from build123d import *

# Parameters (mm, degrees)
SKETCH_W     = 46
SKETCH_H     = 43.5
SKETCH_R     = 18.2
PAD_DEPTH    = 5
SKETCH006_R  = 1.5
POCKET_DEPTH = 5.001
FILLET_R     = 5
FILLET001_R  = 5


with BuildPart() as part:
    # Sketch → Pad (new body)
    with BuildSketch(Plane.YZ):
        with Locations((20, 15.75)):
            Rectangle(SKETCH_W, SKETCH_H)
        with Locations((18.5, 15.75)):
            Circle(SKETCH_R, mode=Mode.SUBTRACT)
    extrude(amount=PAD_DEPTH)

    # Sketch006 → Pocket (cut, through all)
    with BuildSketch(Plane.YZ.offset(5)):
        with Locations((3, 34.5)):
            Circle(SKETCH006_R)
        with Locations((34, 34.5)):
            Circle(SKETCH006_R)
        with Locations((40, 15.75)):
            Circle(SKETCH006_R)
        with Locations((34, -3)):
            Circle(SKETCH006_R)
        with Locations((3, -3)):
            Circle(SKETCH006_R)
    extrude(amount=-POCKET_DEPTH, mode=Mode.SUBTRACT)

    # Fillet
    fillet_edges = [part.edges().sort_by_distance(p)[0] for p in [
        (2.5, 43, -6),
        (2.5, -3, -6),
    ]]
    fillet(fillet_edges, radius=FILLET_R)

    # Fillet001
    fillet001_edges = [part.edges().sort_by_distance(p)[0] for p in [
        (2.5, 43, 37.5),
        (2.5, -3, 37.5),
    ]]
    fillet(fillet001_edges, radius=FILLET001_R)


solid = part.part
Build history of the part. All positions in model axes, mm. Round coordinates to 2 decimals unless told otherwise and drop trailing zeros. Write each loop counter-clockwise with the first axis right and the second up, starting at its lowest first coordinate (ties: lowest second). Pieces come first, ordered by that corner, then holes. Notation, with made-up numbers: (-27, 39.5) -> (27, 39.5) arc R24 ccw to (27, 52.5) -> close; hole circle Ø4 at (-8, -16). An arc over 180 degrees is marked (long way). Use one line per item in the form item = value.
Q1. Drill centre lines: L1, parallel to Z at x = 3.7, y = 18.5; L2, parallel to Z at x = 3.95, y = 3; L3, parallel to Y at x = 0.2, z = 16. Where is each one in solid material? Low to high.
Conclusion:
L1 = -6 to -2.45, 33.95 to 37.5
L2 = -6 to -4.5, -1.5 to 6.21, 25.29 to 33, 36 to 37.5
L3 = -3 to 0.3, 36.7 to 38.52, 41.48 to 43
Q2. Band-saw the part on A-A, the plane y = 18.5. Write the cut outline in (x, z).
Conclusion:
outline = (0, -6) -> (5, -6) -> (5, -2.45) -> (0, -2.45) -> close; (0, 33.95) -> (5, 33.95) -> (5, 37.5) -> (0, 37.5) -> close
Q3. Band-saw the part on B-B, the plane x = 4.4. Write the cut outline in (y, z), then the cut area to 3 significant figures.
Conclusion:
outline = (-3, -1) arc R5 ccw to (2, -6) -> (38, -6) arc R5 ccw to (43, -1) -> (43, 32.5) arc R5 ccw to (38, 37.5) -> (2, 37.5) arc R5 ccw to (-3, 32.5) -> close; hole circle Ø36.4 at (18.5, 15.75); hole circle Ø3 at (3, -3); hole circle Ø3 at (3, 34.5); hole circle Ø3 at (34, -3); hole circle Ø3 at (34, 34.5); hole circle Ø3 at (40, 15.75)
area = 904 mm²
Q4. Two-plate mould, pull along Y, no slides. Class faces 1 (the cylindrical face through (3, 3, 33)), 2 (the cylindrical face through (3, 41, -5)), 3 (the flat face through (2, 20, -6)), 4 (the cylindrical face through (2.54, 32.5, -2.93)): released by +Y, released by -Y, zero draft, split by the parting line, or undercut.
Conclusion:
face_1 = undercut
face_2 = released by +Y
face_3 = zero draft
face_4 = undercut
Q5. Band-saw the part on D-D, the plane z = 34.5. Write the cut outline in (x, y), then the cut area to 3 significant figures.
Conclusion:
outline = (0, -2.58) -> (5, -2.58) -> (5, 1.5) -> (0, 1.5) -> close; (0, 4.5) -> (5, 4.5) -> (5, 32.5) -> (0, 32.5) -> close; (0, 35.5) -> (5, 35.5) -> (5, 42.58) -> (0, 42.58) -> close
area = 196 mm²
Q6. Band-saw the part on C-C, the plane z = 10. Write the cut outline in (x, y), then the cut area to 3 significant figures.
Conclusion:
outline = (0, -3) -> (5, -3) -> (5, 1.23) -> (0, 1.23) -> close; (0, 35.77) -> (5, 35.77) -> (5, 43) -> (0, 43) -> close
area = 57.3 mm²
